Geometry check sheet. Reference: the model listing, model coordinates, mm. Give positions to 0.01 mm unless a question says otherwise; leave off trailing zeros. Loops run counter-clockwise (first coordinate to the right, second up) from the corner with the lowest first, then second, coordinate; pieces in that order, holes last. Notation, with made-up numbers: (66, 0) -> (75, 0) arc R32 cw to (75, 33) -> close; hole circle Ø10 at (50, -34.75). An arc over 180 degrees is marked (long way). Write each question's results on one line, items separated by ' | '. Start each with the question number.
1) Sectioned sample at B-B on x = -55. Record the cut outline in (y, z), then the cut area to 3 significant figures.
2) Sectioned sample at C-C on y = 1.5. Record the cut outline in (x, z).
3) Scan lines: line 1 (Z direction, x = 55, y = 2.95); line 2 (X direction, y = 0.5, z = -7); line 3 (X direction, y = 3.95, z = -7.75). Record each from-to range of solid material in increasing order. Write a range as from..to.
4) Draft check along Z on faces 1 (the face through (-51.185, 2.535, 3.799)), 2 (the face through (-1, 2, -15)), 3 (the face through (51.185, 2.535, -3.799)), 4 (the face through (-65, 2, 0)). Enter one of: pulls with the +Z half, pulls with the -Z half, needs draft (parallel to the pull), parting line crosses it, or undercut.
5) Sectioned sample at A-A on z = 5. Record the cut outline in (x, y).
Autodesk Inventor part; units mm, degrees
ref_plane "Work Plane1" through (0, 39.345, 0) normal (0, 1, 0) x (1, 0, 0)
ref_plane "YZ Plane" through (0, 0, 0) normal (1, 0, 0) x (0, 1, 0)
ref_plane "XZ Plane" through (0, 0, 0) normal (0, 1, 0) x (-1, 0, 0)
sketch "Sketch1" plane through (0, 0, 0) normal (0, 1, 0) x (-1, 0, 0)
  line L0 (-65, 15) -> (65, 15)
  line L1 (65, 15) -> (65, -15)
  line L2 (65, -15) -> (-65, -15)
  line L3 (-65, -15) -> (-65, 15)
  line L4 (-65, 15) -> (65, -15) construction
  line L5 (65, 15) -> (-65, -15) construction
  point P0 (0, 0)
  dimension "d0" = 130
  dimension "d1" = 30
extrude "Plate1" add sketch "Sketch1" along normal blind 5
sketch "Sketch3" plane through (0, 5, 0) normal (0, 1, 0) x (1, 0, 0)
  line L0 (-65, -15) -> (-65, 15)
  line L1 (-65, 0) -> (-55, 0)
  line L2 (-40.6549, -15) -> (-40.6549, 15)
  line L3 (-57.1441, -5) -> (-52.8559, -5)
  line L4 (-52.8559, -5) -> (-52.8559, 5)
  line L5 (-52.8559, 5) -> (-57.1441, 5)
  line L6 (-57.1441, 5) -> (-57.1441, -5)
  line L7 (-57.1441, -5) -> (-52.8559, 5) construction
  line L8 (-52.8559, -5) -> (-57.1441, 5) construction
  circle A0 centre (-55, 5) radius 4
  circle A1 centre (-55, -5) radius 4
  point P0 (0, 0)
  dimension "d10" = 10
  dimension "d11" = 10
  dimension "d12" = 8
  dimension "d13" = 8
extrude "Cut1" cut sketch "Sketch3" against normal blind 5 contours L6 A1 L4 L3 | L3 L4 A1 L6 | A0 L6 L5 L4 | L4 L5 L6 A0
ref_plane "Work Plane1" through (0, 39.345, 0) normal (0, 1, 0) x (1, 0, 0)
mirror "Mirror1" about plane through (0, 39.345, 0) normal (0, 1, 0) of "Cut1"
sketch "Sketch8" plane through (65, 5, 15) normal (0, 1, 0) x (-1, 0, 0)
  circle A0 centre (10, -10) radius 4
  circle A1 centre (10, -10) radius 4
  circle A2 centre (10, -20) radius 4
  circle A3 centre (10, -20) radius 4
  point P0 (65, -15)
extrude "Cut4" cut sketch "Sketch8" against normal blind 5
sketch "Sketch9" plane through (65, 0, -15) normal (0, -1, 0) x (-1, 0, 0)
  point P0 (65, -15)
equation "\"d14\" = Thickness"
equation "\"d36\" = Thickness"
equation "\"d2\" = Thickness"
equation "\"BendRadius\" = Thickness"
equation "\"BendReliefWidth\" = Thickness"
equation "\"BendReliefDepth\" = 0.5 * Thickness"
equation "\"TransitionRadius\" = BendRadius"
equation "\"JacobiRadiusSize\" = BendRadius"
equation "\"GapSize\" = Thickness"
properties part number "up bracket1111" material "Steel, Alloy"
Result:
1) outline: (0, -15) -> (5, -15) -> (5, -9) -> (0, -9) -> close; (0, -1) -> (5, -1) -> (5, 1) -> (0, 1) -> close; (0, 9) -> (5, 9) -> (5, 15) -> (0, 15) -> close | area: 70.0 mm^2
2) outline: (-65, -15) -> (65, -15) -> (65, 15) -> (-65, 15) -> close; hole circle Ø8 at (-55, -5); hole circle Ø8 at (-55, 5); hole circle Ø8 at (55, -5); hole circle Ø8 at (55, 5)
3) line 1: -15..-9, -1..1, 9..15 | line 2: -65..-58.46, -51.54..51.54, 58.46..65 | line 3: -65..-57.9, -52.1..52.1, 57.9..65
4) face 1: undercut | face 2: pulls with the -Z half | face 3: undercut | face 4: needs draft
5) outline: (-65, 0) -> (-59, 0) -> (-59, 5) -> (-65, 5) -> close; (-51, 0) -> (51, 0) -> (51, 5) -> (-51, 5) -> close; (59, 0) -> (65, 0) -> (65, 5) -> (59, 5) -> close
